For this review, take the finished solid that the model builds, in its own axes (mm). A direction names the side the tool comes from. Round coordinates to 2 decimals unless told otherwise and drop trailing zeros. Loops run counter-clockwise (first coordinate to the right, second up) from the corner with the lowest first, then second, coordinate; pieces in that order, holes last. Notation, with made-up numbers: (40, -4.5) -> (88, -4.5) arc R29 cw to (88, 25.5) -> close; hole circle Ø6 at (-12.5, 10.5). An arc over 180 degrees is marked (long way). One line per question, with ' | ' between items. Start each with the question number.
1. Consider section C-C (z = -2.5). Write out the cut boundary in (x, y), and give its area (3 significant figures).
2. Consider section D-D (x = 0). Write out the cut boundary in (y, z), and give its area (3 significant figures).
3. For faces 1 (the face through (0, 3.9, -21)), 2 (the face through (6.5, 11, -6)), 3 (the face through (-22.414, 1.014, 5.292)), 4 (the face through (-20, 2, 0)), 5 (the face through (-20, 1, -8.5)), list the 3-axis set-ups (+Z, -Z, +X, -X, +Y, -Y) from which the entire face can be reached by the end or side of a thin tool; tool diameter is ignored.
4. For pin 1 Ø4 at (y, z) = (16, -16.5) entering from -X; pin 2 Ø5 at (y, z) = (6.5, -12) entering from +X; pin 3 Ø4 at (x, z) = (24, 5.5) entering from +Y, all flat-tipped, find the tip position at first contact; note any pin that passes through.
5. Consider section A-A (x = 24). Write out the cut boundary in (y, z).
6. Draft analysis for pull direction Z (two halves, no side actions). For faces 6 (the face through (0.225, 17.66, -20.385)), 7 (the face through (20, 1, -8.5)), 8 (the face through (25.586, 1.014, 5.292)), 9 (the face through (7, 18.4, -9)), state which applies: pulls with the +Z half, pulls with the -Z half, needs draft (parallel to the pull), parting line crosses it, or undercut.
7. Consider section B-B (y = 7.5). Write out the cut boundary in (x, z), and give its area (3 significant figures).
8. Wall thickness on line 1 along X through (y, z) = (1.15, 5.5); line 2 along X through (y, z) = (15.75, 4.5); line 3 along X through (y, z) = (17.7, -21.1): over which ranges is each line inside the solid? List them lowest first.
```python
from build123d import *

# Parameters (mm, degrees)
SKETCH1_W           = 60
SKETCH1_H           = 17
BOSS_EXTRUDE1_DEPTH = 4
SKETCH4_W           = 19
SKETCH4_H           = 4
BOSS_EXTRUDE2_DEPTH = 14
SKETCH5_W           = 3
SKETCH5_H           = 31
BOSS_EXTRUDE3_DEPTH = 14.4
SKETCH6_W           = 13
SKETCH6_H           = 2.5
BOSS_EXTRUDE4_DEPTH = 14.4
SKETCH7_W           = 9
SKETCH7_H           = 2.5
CUT_EXTRUDE1_DEPTH  = 14.4
SKETCH8_W           = 13
SKETCH8_H           = 3
BOSS_EXTRUDE5_DEPTH = 14.4
SKETCH9_R           = 0.75
CUT_EXTRUDE2_DEPTH  = 6
SKETCH10_W          = 10
SKETCH10_H          = 8
CUT_EXTRUDE3_DEPTH  = 3
FILLET1_R           = 1
SKETCH11_R          = 1.6
CUT_EXTRUDE4_DEPTH  = 4
SKETCH12_W          = 20.5
SKETCH12_H          = 17
CUT_EXTRUDE5_DEPTH  = 2
SKETCH13_W          = 10
SKETCH13_H          = 3
CUT_EXTRUDE6_DEPTH  = 5


with BuildPart() as part:
    # Sketch1 → Boss-Extrude1 (new body)
    with BuildSketch(Plane(origin=(0, 0, 0), x_dir=(1, 0, 0), z_dir=(0, 1, 0))):
        Rectangle(SKETCH1_W, SKETCH1_H)
    extrude(amount=BOSS_EXTRUDE1_DEPTH)

    # Sketch4 → Boss-Extrude2 (add)
    with BuildSketch(Plane(origin=(0, 0, -8.5), x_dir=(-1, 0, 0), z_dir=(0, 0, -1))):
        with Locations((0, 2)):
            Rectangle(SKETCH4_W, SKETCH4_H)
    extrude(amount=BOSS_EXTRUDE2_DEPTH)

    # Sketch5 → Boss-Extrude3 (add)
    with BuildSketch(Plane(origin=(0, 4, 0), x_dir=(1, 0, 0), z_dir=(0, 1, 0))):
        with Locations((-8, 7)):
            Rectangle(SKETCH5_W, SKETCH5_H)
    boss_extrude3 = extrude(amount=BOSS_EXTRUDE3_DEPTH)

    # Mirror1: Boss-Extrude3 across plane
    add(boss_extrude3.mirror(Plane(origin=(0, 0, 0), x_dir=(0, 0, 1), z_dir=(1, 0, 0))))

    # Sketch6 → Boss-Extrude4 (add)
    with BuildSketch(Plane(origin=(0, 4, 0), x_dir=(1, 0, 0), z_dir=(0, 1, 0))):
        with Locations((0, -7.25)):
            Rectangle(SKETCH6_W, SKETCH6_H)
    extrude(amount=BOSS_EXTRUDE4_DEPTH)

    # Sketch7 → Cut-Extrude1 (cut)
    with BuildSketch(Plane(origin=(0, 18.4, 0), x_dir=(1, 0, 0), z_dir=(0, 1, 0))):
        with Locations((0, -7.25)):
            Rectangle(SKETCH7_W, SKETCH7_H)
    extrude(amount=-CUT_EXTRUDE1_DEPTH, mode=Mode.SUBTRACT)

    # Sketch8 → Boss-Extrude5 (add)
    with BuildSketch(Plane(origin=(0, 4, 0), x_dir=(1, 0, 0), z_dir=(0, 1, 0))):
        with Locations((0, 21)):
            Rectangle(SKETCH8_W, SKETCH8_H)
    extrude(amount=BOSS_EXTRUDE5_DEPTH)

    # Sketch9 → Cut-Extrude2 (cut)
    with BuildSketch(Plane(origin=(0, 18.4, 0), x_dir=(1, 0, 0), z_dir=(0, 1, 0))):
        with Locations(Location((0, 21.1, 0), (0, 0, 270))):
            Circle(SKETCH9_R)
    extrude(amount=-CUT_EXTRUDE2_DEPTH, mode=Mode.SUBTRACT)

    # Sketch10 → Cut-Extrude3 (cut)
    with BuildSketch(Plane(origin=(0, 0, -22.5), x_dir=(-1, 0, 0), z_dir=(0, 0, -1))):
        with Locations((0, 12.9)):
            Rectangle(SKETCH10_W, SKETCH10_H)
    extrude(amount=-CUT_EXTRUDE3_DEPTH, mode=Mode.SUBTRACT)

    # Fillet1
    fillet1_edges = [part.edges().sort_by_distance(p)[0] for p in [
        (-6.5, 11.2, -19.5),
        (6.5, 11.2, -19.5),
    ]]
    fillet(fillet1_edges, radius=FILLET1_R)

    # Sketch11 → Cut-Extrude4 (cut)
    with BuildSketch(Plane(origin=(0, 4, 0), x_dir=(1, 0, 0), z_dir=(0, 1, 0))):
        with Locations(Location((-24, -5.5, 0), (0, 0, 270))):
            Circle(SKETCH11_R)
        with Locations(Location((24, -5.5, 0), (0, 0, 270))):
            Circle(SKETCH11_R)
    extrude(amount=-CUT_EXTRUDE4_DEPTH, mode=Mode.SUBTRACT)

    # Sketch12 → Cut-Extrude5 (cut)
    with BuildSketch(Plane(origin=(0, 4, 0), x_dir=(1, 0, 0), z_dir=(0, 1, 0))):
        with Locations((-19.75, 0)):
            Rectangle(SKETCH12_W, SKETCH12_H)
    cut_extrude5 = extrude(amount=-CUT_EXTRUDE5_DEPTH, mode=Mode.SUBTRACT)

    # Mirror2: Cut-Extrude5 across plane
    add(cut_extrude5.mirror(Plane(origin=(0, 0, 0), x_dir=(0, 0, 1), z_dir=(1, 0, 0))), mode=Mode.SUBTRACT)

    # Sketch13 → Cut-Extrude6 (cut)
    with BuildSketch(Plane(origin=(0, 8.9, 0), x_dir=(1, 0, 0), z_dir=(0, 1, 0))):
        with Locations((0, 21)):
            Rectangle(SKETCH13_W, SKETCH13_H)
    extrude(amount=-CUT_EXTRUDE6_DEPTH, mode=Mode.SUBTRACT)


solid = part.part
```
Answer block:
1) outline: (-30, 0) -> (30, 0) -> (30, 2) -> (9.5, 2) -> (9.5, 18.4) -> (6.5, 18.4) -> (6.5, 4) -> (-6.5, 4) -> (-6.5, 18.4) -> (-9.5, 18.4) -> (-9.5, 2) -> (-30, 2) -> close | area: 244 mm2
2) outline: (0, -22.5) -> (3.9, -22.5) -> (3.9, -19.5) -> (4, -19.5) -> (4, 8.5) -> (0, 8.5) -> close; (16.9, -22.5) -> (18.4, -22.5) -> (18.4, -21.85) -> (16.9, -21.85) -> close; (16.9, -20.35) -> (18.4, -20.35) -> (18.4, -19.5) -> (16.9, -19.5) -> close | area: 126 mm2
3) face 1: -Z | face 2: +Y | face 3: +Y, -Y | face 4: +Z, -Z, -X, +Y | face 5: -Z, -X, +Y, -Y
4) pin 1: stops at x = -9.5 | pin 2: stops at x = 9.5 | pin 3: stops at y = 2
5) outline: (0, -8.5) -> (2, -8.5) -> (2, 3.9) -> (0, 3.9) -> close; (0, 7.1) -> (2, 7.1) -> (2, 8.5) -> (0, 8.5) -> close
6) face 6: undercut | face 7: pulls with the -Z half | face 8: undercut | face 9: needs draft
7) outline: (-9.5, -22.5) -> (-5, -22.5) -> (-5, -19.5) -> (-5.5, -19.5) arc R1 cw to (-6.5, -18.5) -> (-6.5, 6) -> (-4.5, 6) -> (-4.5, 8.5) -> (-9.5, 8.5) -> close; (4.5, 6) -> (6.5, 6) -> (6.5, -18.5) arc R1 cw to (5.5, -19.5) -> (5, -19.5) -> (5, -22.5) -> (9.5, -22.5) -> (9.5, 8.5) -> (4.5, 8.5) -> close | area: 205 mm2
8) line 1: x = -30 to -25.6, -22.4 to 22.4, 25.6 to 30 | line 2: x = -9.5 to -6.5, 6.5 to 9.5 | line 3: x = -9.5 to -0.75, 0.75 to 9.5
